from build123d import *

# Parameters (mm, degrees)
CYLINDER005_R           = 1.4
CYLINDER005_DEPTH       = 18
CYLINDER005_ROLL_ANGLE  = 90
CYLINDER012_R           = 1.4
CYLINDER012_DEPTH       = 18
CYLINDER012_PITCH_ANGLE = 90
CYLINDER004_R           = 5.7
CYLINDER004_DEPTH       = 6
CHAMFER_SIZE            = 1


with BuildPart() as cylinder005:
    # Cylinder005 → Cylinder005 (new body)
    with BuildSketch(Plane.XY):
        Circle(CYLINDER005_R)
    extrude(amount=CYLINDER005_DEPTH)


with BuildPart() as cylinder005_1:
    # Cylinder005 roll: moved
    add(cylinder005.part.rotate(Axis((0, 0, 0), (1, 0, 0)), CYLINDER005_ROLL_ANGLE))


with BuildPart() as cylinder005_2:
    # Cylinder005 placement: moved
    add(cylinder005_1.part.moved(Location((0, 9, 3))))


with BuildPart() as joiner_pins:
    # Cylinder012 → Cylinder012 (new body)
    with BuildSketch(Plane.XY):
        Circle(CYLINDER012_R)
    extrude(amount=CYLINDER012_DEPTH)


with BuildPart() as joiner_pins_1:
    # Cylinder012 pitch: moved
    add(joiner_pins.part.rotate(Axis((0, 0, 0), (0, 1, 0)), CYLINDER012_PITCH_ANGLE))


with BuildPart() as joiner_pins_2:
    # Cylinder012 placement: moved
    add(joiner_pins_1.part.moved(Location((-9, 0, 3))))

    # Fusion002: union Cylinder005
    add(cylinder005_2.part)


with BuildPart() as joiner:
    # Cylinder004 → Cylinder004 (new body)
    with BuildSketch(Plane.XY):
        Circle(CYLINDER004_R)
    extrude(amount=CYLINDER004_DEPTH)

    # Cut009: cut joiner pins
    add(joiner_pins_2.part, mode=Mode.SUBTRACT)

    # Chamfer
    chamfer_edges = [joiner.edges().sort_by_distance(p)[0] for p in [
        (-5.7, 0, 0),
        (-5.7, 0, 6),
    ]]
    chamfer(chamfer_edges, length=CHAMFER_SIZE)


with BuildPart() as joiner_1:
    # Chamfer placement: moved
    add(joiner.part.moved(Location((20, 0, 0))))


solid = joiner_1.part
The model under review builds one solid part; all positions refer to its coordinate system, in mm. Coordinates: 2 decimals unless noted, no trailing zeros. Write each loop counter-clockwise with the first axis right and the second up, starting at its lowest first coordinate (ties: lowest second). Pieces come first, ordered by that corner, then holes. Notation, with made-up numbers: (-22, 52.5) -> (-2, 52.5) arc R23 ccw to (-2, 74.5) -> close; hole circle Ø5 at (37.25, 37). An arc over 180 degrees is marked (long way). Answer in a Markdown table with one row per item.
1. Draft analysis for pull direction Z (two halves, no side actions). For faces 1 (the flat face through (20, 0, 0)), 2 (the cylindrical face through (23.44, -0.85, 4.11)), 3 (the flat face through (20, 0, 6)), state which applies: +Z half, -Z half, draft (parallel to the pull), parting line (faces both ways), or undercut.
Answers below:
| item | result |
|---|---|
| face 1 | -Z half |
| face 2 | undercut |
| face 3 | +Z half |
2. We need section A-A, the plane z = 4.2. State the section outline as (x, y) points.
Answers below:
| item | result |
|---|---|
| outline | (14.35, -0.72) arc R5.7 ccw to (19.28, -5.65) -> (19.28, -0.72) -> close; (14.35, 0.72) -> (19.28, 0.72) -> (19.28, 5.65) arc R5.7 ccw to start; (20.72, -5.65) arc R5.7 ccw to (25.65, -0.72) -> (20.72, -0.72) -> close; (20.72, 0.72) -> (25.65, 0.72) arc R5.7 ccw to (20.72, 5.65) -> close |
3. We need section B-B, the plane z = 3. State the section outline as (x, y) points, and give its area (3 significant figures).
Answers below:
| item | result |
|---|---|
| outline | (14.47, -1.4) arc R5.7 ccw to (18.6, -5.53) -> (18.6, -1.4) -> close; (14.47, 1.4) -> (18.6, 1.4) -> (18.6, 5.53) arc R5.7 ccw to start; (21.4, -5.53) arc R5.7 ccw to (25.53, -1.4) -> (21.4, -1.4) -> close; (21.4, 1.4) -> (25.53, 1.4) arc R5.7 ccw to (21.4, 5.53) -> close |
| area | 46.7 mm^2 |
4. Clearance check with flat-ended pins moving along their axes: pin 1 Ø3 at (y, z) = (0, 3) entering from +X; pin 2 Ø2 at (x, z) = (18, 4) entering from -Y; pin 3 Ø1 at (y, z) = (4, 4.5) entering from +X. State where each tip first meets the part, or that it passes through.
Answers below:
| item | result |
|---|---|
| pin 1 | stops at x = 25.7 |
| pin 2 | stops at y = -5.61 |
| pin 3 | stops at x = 24.5 |
5. Wall thickness on probe 1 along Z at (x, y) = (22.5, 0); probe 2 along Y at (x, z) = (15.95, 3); probe 3 along X at (y, z) = (-3.5, 1.9): over which ranges is each line inside the solid? List them lowest first. Write a range as [from, to].
Answers below:
| item | result |
|---|---|
| probe 1 | z = [0, 1.6], [4.4, 6] |
| probe 2 | y = [-4.01, -1.4], [1.4, 4.01] |
| probe 3 | x = [15.5, 19.13], [20.87, 24.5] |
